Geometry check sheet. Reference: the model listing, model coordinates, mm. Face numbers are marked on the shaded views. Coordinates: 2 decimals unless noted, no trailing zeros. Write each loop counter-clockwise with the first axis right and the second up, starting at its lowest first coordinate (ties: lowest second). Pieces come first, ordered by that corner, then holes. Notation, with made-up numbers: (89, -5.75) -> (142, -5.75) arc R31 cw to (142, 25.25) -> close; hole circle Ø1 at (69, -28.5). An arc over 180 degrees is marked (long way). One line per question, with ' | ' between items.
from build123d import *

# Parameters (mm, degrees)
F0_W     = 400
F0_H     = 800
F1_DEPTH = 100
F2_SIZE  = 50
F3_R     = 25
F4_R     = 50
F5_DEPTH = 230


with BuildPart() as f1:
    # F0 (on Front) → F1 (new body, symmetric)
    with BuildSketch(Plane.XZ):
        Rectangle(F0_W, F0_H)
    extrude(amount=F1_DEPTH, both=True)

    # F2
    f2_edges = [f1.edges().sort_by_distance(p)[0] for p in [
        (-200, 0, 400),
        (200, 0, 400),
    ]]
    chamfer(f2_edges, length=F2_SIZE)

    # F3
    f3_edges = [f1.edges().sort_by_distance(p)[0] for p in [
        (-200, 0, -400),
        (200, 0, -400),
    ]]
    fillet(f3_edges, radius=F3_R)

    # F4 (on face) → F5 (cut)
    with BuildSketch(Plane.XZ.offset(100)):
        Circle(F4_R)
    extrude(amount=-F5_DEPTH, mode=Mode.SUBTRACT)


solid = f1.part
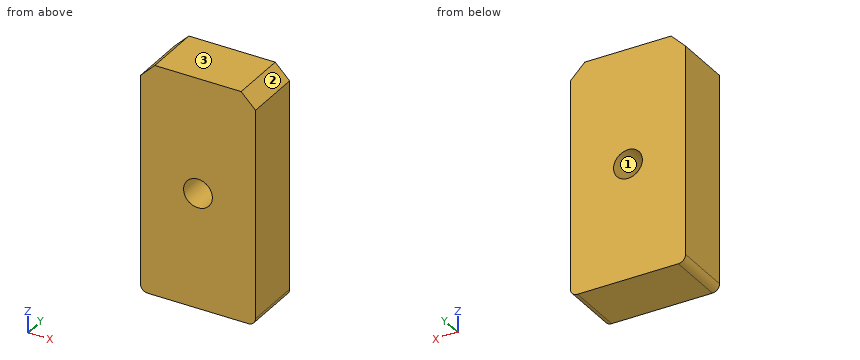
1. Material ranges on line 1 (Z direction, x = 0, y = 1); line 2 (Z direction, x = 16, y = -84); line 3 (Z direction, x = 163.5, y = 83.5), recorded low to high. Write a range as from..to.
Worked answers:
line 1: -400..-50, 50..400 | line 2: -400..-47.37, 47.37..400 | line 3: -400..386.5
2. Cross-section at B-B on y = 65.5. Record the boundary of the cut face in (x, z).
Worked answers:
outline: (-200, -375) arc R25 ccw to (-175, -400) -> (175, -400) arc R25 ccw to (200, -375) -> (200, 350) -> (150, 400) -> (-150, 400) -> (-200, 350) -> close; hole circle Ø100 at (0, 0)
3. Cross-section at A-A on x = 0. Record the boundary of the cut face in (y, z).
Worked answers:
outline: (-100, -400) -> (100, -400) -> (100, -50) -> (-100, -50) -> close; (-100, 50) -> (100, 50) -> (100, 400) -> (-100, 400) -> close
4. Mould release check, pull along X, two halves, no side actions. Record for the marked faces 1, 2 and 3: released by +X, released by -X, zero draft, split by the parting line, or undercut.
Worked answers:
face 1: undercut | face 2: released by +X | face 3: zero draft
5. Cross-section at C-C on z = 0. Record the boundary of the cut face in (x, y), and give its area (3 significant figures).
Worked answers:
outline: (-200, -100) -> (-50, -100) -> (-50, 100) -> (-200, 100) -> close; (50, -100) -> (200, -100) -> (200, 100) -> (50, 100) -> close | area: 60,000 mm²
